Autodesk Inventor part; units mm, degrees
ref_plane "YZ Plane" through (0, 0, 0) normal (1, 0, 0) x (0, 1, 0)
ref_plane "XZ Plane" through (0, 0, 0) normal (0, 1, 0) x (-1, 0, 0)
ref_plane "XY Plane" through (0, 0, 0) normal (0, 0, 1) x (1, 0, 0)
sketch "Sketch1" plane through (0, 0, 0) normal (0, 0, 1) x (1, 0, 0)
  line L0 (80, 30) -> (-80, 30)
  line L1 (-80, 30) -> (-80, -30)
  line L2 (-80, -30) -> (80, -30)
  line L3 (80, -30) -> (80, 30)
  line L4 (80, 30) -> (-80, -30) construction
  line L5 (-80, 30) -> (80, -30) construction
  line L6 (-20, -30) -> (-80, -30)
  line L7 (-80, -30) -> (-80, 30)
  line L8 (-80, 30) -> (-20, 30)
  line L9 (-20, 30) -> (-20, -30)
  line L10 (-20, -30) -> (-80, 30) construction
  line L11 (-80, -30) -> (-20, 30) construction
  line L12 (20, -30) -> (80, -30)
  line L13 (80, -30) -> (80, 30)
  line L14 (80, 30) -> (20, 30)
  line L15 (20, 30) -> (20, -30)
  line L16 (20, -30) -> (80, 30) construction
  line L17 (80, -30) -> (20, 30) construction
  line L18 (0, 30) -> (0, -30) construction
  point P0 (0, 0)
  point P1 (-50, 0)
  point P2 (50, 0)
  point P3 (20, 30)
  point P4 (20, -30)
  point P5 (-20, -30)
  point P6 (-20, 30)
  dimension "d0" = 160
  dimension "d1" = 60
  dimension "d2" = 40
extrude "Extrusion1" add sketch "Sketch1" along normal blind 10 contours L3 L2 L15 L0 | L9 L2 L1 L0
sketch "Sketch2" plane through (0, 0, 10) normal (0, 0, 1) x (1, 0, 0)
  line L0 (-80, -30) -> (-20, -30)
  line L1 (80, -24) -> (-80, -24)
  line L2 (-80, -24) -> (-80, -30)
  line L3 (-80, -30) -> (80, -30)
  line L4 (80, -30) -> (80, -24)
  line L5 (80, -24) -> (-80, -30) construction
  line L6 (-80, -24) -> (80, -30) construction
  line L7 (80, -30) -> (80, 30)
  point P0 (0, 0)
  point P1 (0, -27)
  dimension "d5" = 6
extrude "Extrusion2" add sketch "Sketch2" along normal blind 115
sketch "Sketch3" plane through (0, 0, 0) normal (0, 0, -1) x (-1, 0, 0)
  line L0 (53, 7.5) -> (43, 7.5)
  line L1 (43, 7.5) -> (43, -7.5)
  line L2 (43, -7.5) -> (53, -7.5)
  line L3 (53, -7.5) -> (53, 7.5)
  line L4 (53, 7.5) -> (43, -7.5) construction
  line L5 (43, 7.5) -> (53, -7.5) construction
  line L6 (-43, 7.5) -> (-53, 7.5)
  line L7 (-53, 7.5) -> (-53, -7.5)
  line L8 (-53, -7.5) -> (-43, -7.5)
  line L9 (-43, -7.5) -> (-43, 7.5)
  line L10 (-43, 7.5) -> (-53, -7.5) construction
  line L11 (-53, 7.5) -> (-43, -7.5) construction
  line L12 (80, -30) -> (-80, -30) construction
  line L13 (0, -30) -> (0, 0) construction
  point P0 (48, 0)
  point P1 (-48, 0)
  point P2 (48, 0)
  dimension "d8" = 10
  dimension "d9" = 15
  dimension "d10" = 48
extrude "Extrusion3" cut sketch "Sketch3" against normal through all
sketch "Sketch4" plane through (0, 0, 0) normal (0, 0, -1) x (-1, 0, 0)
  line L0 (-70, -20) -> (70, -20) construction
  line L1 (70, -20) -> (70, 20) construction
  line L2 (70, 20) -> (-70, 20) construction
  line L3 (-70, 20) -> (-70, -20) construction
  line L4 (-70, -20) -> (70, 20) construction
  line L5 (70, -20) -> (-70, 20) construction
  circle A0 centre (70, 20) radius 1.25
  circle A1 centre (-70, 20) radius 1.25
  circle A2 centre (-70, -20) radius 1.25
  circle A3 centre (70, -20) radius 1.25
  line L6 (40, -20) -> (-40, -20) construction
  line L7 (-40, -20) -> (-40, 20) construction
  line L8 (-40, 20) -> (40, 20) construction
  line L9 (40, 20) -> (40, -20) construction
  line L10 (40, -20) -> (-40, 20) construction
  line L11 (-40, -20) -> (40, 20) construction
  circle A4 centre (-40, 20) radius 1.25
  circle A5 centre (-40, -20) radius 1.25
  circle A6 centre (40, 20) radius 1.25
  circle A7 centre (40, -20) radius 1.25
  point P0 (0, 0)
  dimension "d13" = 140
  dimension "d14" = 40
  dimension "d16" = 2.5
  dimension "d54" = 80
extrude "Extrusion4" cut sketch "Sketch4" against normal through all
sketch "Sketch5" plane through (-20, -24, 10) normal (0, 1, 0) x (1, 0, 0)
  line L0 (59.5, -13) -> (-19.5, -13) construction
  line L1 (-19.5, -13) -> (-19.5, -113) construction
  line L2 (-19.5, -113) -> (59.5, -113) construction
  line L3 (59.5, -113) -> (59.5, -13) construction
  line L4 (59.5, -13) -> (-19.5, -113) construction
  line L5 (-19.5, -13) -> (59.5, -113) construction
  line L6 (100, -115) -> (-60, -115) construction
  line L7 (55.5, -17) -> (-2.5, -17) construction
  line L8 (-2.5, -17) -> (-2.5, -103) construction
  line L9 (-2.5, -103) -> (55.5, -103) construction
  line L10 (55.5, -103) -> (55.5, -17) construction
  line L11 (55.5, -17) -> (-2.5, -103) construction
  line L12 (-2.5, -17) -> (55.5, -103) construction
  circle A0 centre (-2.5, -17) radius 1.75
  circle A1 centre (55.5, -17) radius 1.75
  circle A2 centre (-2.5, -103) radius 1.75
  circle A3 centre (55.5, -103) radius 1.75
  line L13 (-60, -22) -> (-24, -22)
  line L14 (-24, -22) -> (-24, -98)
  line L15 (-24, -98) -> (-60, -98)
  line L16 (-60, -98) -> (-60, -22)
  line L17 (-60, -22) -> (-24, -98) construction
  line L18 (-24, -22) -> (-60, -98) construction
  line L19 (100, -22) -> (64, -22)
  line L20 (64, -22) -> (64, -98)
  line L21 (64, -98) -> (100, -98)
  line L22 (100, -98) -> (100, -22)
  line L23 (100, -22) -> (64, -98) construction
  line L24 (64, -22) -> (100, -98) construction
  line L25 (20, 10) -> (20, -115) construction
  line L26 (-60, 0) -> (-60, -115) construction
  circle A4 centre (-42, -16.5) radius 1.25
  circle A5 centre (-42, -103.5) radius 1.25
  circle A6 centre (82, -16.5) radius 1.25
  circle A7 centre (82, -103.5) radius 1.25
  line L27 (-60, 10) -> (-60, -115) construction
  line L28 (0, 0) -> (-60, 0)
  circle A8 centre (-2.5, -17) radius 3
  circle A9 centre (55.5, -17) radius 3
  circle A10 centre (-2.5, -103) radius 3
  circle A11 centre (55.5, -103) radius 3
  point P0 (20, -63)
  point P1 (20, -63)
  point P2 (26.5, -60)
  point P3 (20, -63)
  point P4 (26.5, -60)
  point P5 (-42, -60)
  point P6 (82, -60)
  point P7 (-42, -60)
  point P8 (82, -60)
  point P9 (-42, -60)
  point P10 (82, -60)
  dimension "d20" = 79
  dimension "d21" = 100
  dimension "d22" = 58
  dimension "d23" = 86
  dimension "d26" = 4
  dimension "d27" = 4
  dimension "d28" = 3.5
  dimension "d31" = 36
  dimension "d32" = 76
  dimension "d36" = 2.5
  dimension "d39" = 13
  dimension "d42" = 4.5
  dimension "d45" = 6
  dimension "d50" = 43.5
  dimension "d51" = 43.5
  dimension "d52" = 55
extrude "Extrusion5" cut sketch "Sketch5" against normal through all contours A0 | A1 | A2 | A3
extrude "Extrusion6" cut sketch "Sketch5" against normal through all contours L13 L14 L15 L16 | L22 L21 L20 L19
extrude "Extrusion7" cut sketch "Sketch5" against normal through all contours A4 | A5 | A6 | A7
extrude "Extrusion8" add sketch "Sketch5" along normal blind 4 contours A8 | A9 | A10 | A11
fillet "Fillet1" radius 1 4 edges at (-25.5, -24, 27) (32.5, -24, 27) (-25.5, -24, 113) (32.5, -24, 113)
properties part number "electrical_system_fix_board"
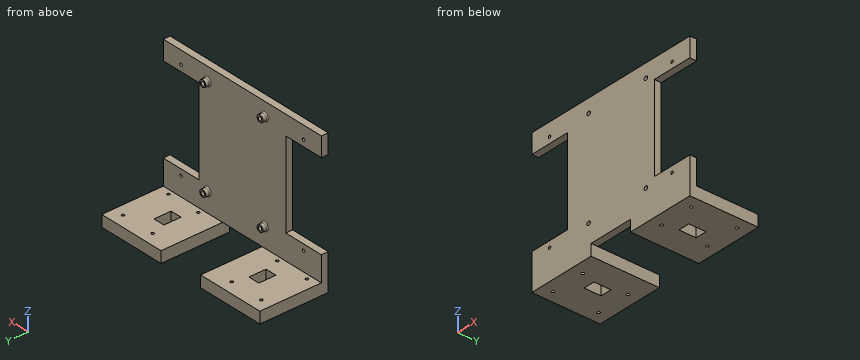
Verification items for the finished model (mm, model axes). Give positions to 0.01 mm unless a question says otherwise; leave off trailing zeros. Loops run counter-clockwise (first coordinate to the right, second up) from the corner with the lowest first, then second, coordinate; pieces in that order, holes last. Notation, with made-up numbers: (-33, 41.5) - (18, 41.5) arc R18 ccw to (18, 70.5) - close; hole circle Ø5 at (44.5, 73.25). An arc over 180 degrees is marked (long way). Write each question's results on one line, items separated by ' | '.
1) Sectioned sample at D-D on x = -22.5. Record the boundary of the cut face in (y, z).
Solution:
outline: (-30, 0) - (30, 0) - (30, 10) - (-24, 10) - (-24, 23) arc R1 cw to (-23, 24) - (-20, 24) - (-20, 25.25) - (-30, 25.25) - close; (-30, 28.75) - (-20, 28.75) - (-20, 30) - (-23, 30) arc R1 cw to (-24, 31) - (-24, 109) arc R1 cw to (-23, 110) - (-20, 110) - (-20, 111.25) - (-30, 111.25) - close; (-30, 114.75) - (-20, 114.75) - (-20, 116) - (-23, 116) arc R1 cw to (-24, 117) - (-24, 125) - (-30, 125) - close
2) Sectioned sample at A-A on y = 1. Record the boundary of the cut face in (x, z).
Solution:
outline: (-80, 0) - (-53, 0) - (-53, 10) - (-80, 10) - close; (-43, 0) - (-20, 0) - (-20, 10) - (-43, 10) - close; (20, 0) - (43, 0) - (43, 10) - (20, 10) - close; (53, 0) - (80, 0) - (80, 10) - (53, 10) - close
3) Depth check by flat-ended pin: P1, Ø3, axis at x = -70, y = -20, coming from the +Z side; P2, Ø1.8, axis at x = -22, z = 112, coming from the +Y side; P3, Ø8, axis at x = -6.5, z = 40, coming from the +Y side. Enter the tip coordinate at first touch or a pass-through.
Solution:
P1: z = 10 | P2: y = -20 | P3: y = -24
4) Sectioned sample at B-B on x = -49.5. Record the boundary of the cut face in (y, z).
Solution:
outline: (-30, 0) - (-7.5, 0) - (-7.5, 10) - (-24, 10) - (-24, 32) - (-30, 32) - close; (-30, 108) - (-24, 108) - (-24, 125) - (-30, 125) - close; (7.5, 0) - (30, 0) - (30, 10) - (7.5, 10) - close
5) Material ranges on L1, parallel to X at y = -22, z = 27; L2, parallel to X at y = -16.5, z = 9; L3, parallel to X at y = -25, z = 113, recorded low to high. Write a range as from..to.
Solution:
L1: -25.5..-24.25, -20.75..-19.5, 32.5..33.75, 37.25..38.5 | L2: -80..-20, 20..80 | L3: -80..-63.15, -60.85..-24.25, -20.75..33.75, 37.25..60.85, 63.15..80
6) Sectioned sample at C-C on y = 15.5. Record the boundary of the cut face in (x, z), plus the area to 3 significant figures.
Solution:
outline: (-80, 0) - (-20, 0) - (-20, 10) - (-80, 10) - close; (20, 0) - (80, 0) - (80, 10) - (20, 10) - close | area: 1,200 mm2
